Design review of the part built by this model. Coordinates are the model's own, in mm. A direction names the side the tool comes from. Give positions to 0.01 mm unless a question says otherwise; leave off trailing zeros. Loops run counter-clockwise (first coordinate to the right, second up) from the corner with the lowest first, then second, coordinate; pieces in that order, holes last. Notation, with made-up numbers: (36, 67.5) - (91, 67.5) arc R37 cw to (91, 103.5) - close; hole circle Ø11 at (-19.5, -35). An arc over 180 degrees is marked (long way). Write each question's results on one line, items separated by ' | '.
```python
from build123d import *

# Parameters (mm, degrees)
F1_DEPTH = 165.1
F3_D     = 25.4
F3_DEPTH = 25.4
F3_TIP   = 7.6309298617


with BuildPart() as f1:
    # F0 (on Right) → F1 (new body)
    with BuildSketch(Plane.YZ):
        Polygon((0, 31.75), (0, 0), (19.05, 0), (19.05, 12.7), (19.05, 31.75), align=None)
        Polygon((19.05, 31.75), (19.05, 12.7), (69.85, 12.7), (69.85, 31.75), (69.85, 44.45), (19.05, 44.45), align=None)
        Polygon((69.85, 12.7), (69.85, 0), (88.9, 0), (88.9, 31.75), (69.85, 31.75), align=None)
    extrude(amount=F1_DEPTH)

    # F3
    with Locations(Plane.XY.offset(44.45)):
        with Locations((130.302, 44.45), (35.052, 44.45)):
            Hole(F3_D / 2, depth=F3_DEPTH)
            with Locations((0, 0, -(F3_DEPTH + F3_TIP / 2))):  # 118° drill point
                Cone(0, F3_D / 2, F3_TIP, mode=Mode.SUBTRACT)


solid = f1.part
```
Item 1: Tool access review of faces 5 (the face through (81, 80, 31.75)), 6 (the face through (29.192, 33.183, 31.572)), 7 (the face through (81, 88.9, 16)), 8 (the face through (81, 10, 31.75)), 9 (the face through (81, 69.85, 6)): name each direction out of +Z, -Z, +X, -X, +Y, -Y from which nothing blocks a thin tool from reaching the whole face with its end or side.
Output values:
face 5: +Z, +X, -X, +Y | face 6: +Z | face 7: +Z, -Z, +X, -X, +Y | face 8: +Z, +X, -X, -Y | face 9: -Z, +X, -X
Item 2: Wall thickness on probe 1 along X at (y, z) = (44.45, 30.75); probe 2 along X at (y, z) = (44, 25); probe 3 along Y at (x, z) = (13, 5.5): over which ranges is each line inside the solid? List them lowest first.
Output values:
probe 1: x = 0 to 22.35, 47.75 to 117.6, 143 to 165.1 | probe 2: x = 0 to 22.36, 47.74 to 117.61, 142.99 to 165.1 | probe 3: y = 0 to 19.05, 69.85 to 88.9
Item 3: We need section D-D on x = 102.5. Give the boundary of the cut face in (y, z).
Output values:
outline: (0, 0) - (19.05, 0) - (19.05, 12.7) - (69.85, 12.7) - (69.85, 0) - (88.9, 0) - (88.9, 31.75) - (69.85, 31.75) - (69.85, 44.45) - (19.05, 44.45) - (19.05, 31.75) - (0, 31.75) - close
Item 4: We need section B-B on y = 44.45. Give the boundary of the cut face in (x, z).
Output values:
outline: (0, 12.7) - (32.92, 12.7) - (22.35, 19.05) - (22.35, 44.45) - (0, 44.45) - close; (37.18, 12.7) - (128.17, 12.7) - (117.6, 19.05) - (117.6, 44.45) - (47.75, 44.45) - (47.75, 19.05) - close; (132.43, 12.7) - (165.1, 12.7) - (165.1, 44.45) - (143, 44.45) - (143, 19.05) - close
Item 5: Draft analysis for pull direction X (two halves, no side actions). For faces 1 (the face through (34.688, 47.219, 13.097)), 2 (the face through (118.57, 39.59, 31.57)), 3 (the face through (81, 79, 0)), 4 (the face through (0, 44, 23)), state which applies: +X half, -X half, draft (parallel to the pull), parting line (faces both ways), or undercut.
Output values:
face 1: undercut | face 2: undercut | face 3: draft | face 4: -X half
Item 6: We need section C-C on z = 26.5. Give the boundary of the cut face in (x, y).
Output values:
outline: (0, 0) - (165.1, 0) - (165.1, 88.9) - (0, 88.9) - close; hole circle Ø25.4 at (35.05, 44.45); hole circle Ø25.4 at (130.3, 44.45)
Item 7: We need section A-A on z = 7. Give the boundary of the cut face in (x, y).
Output values:
outline: (0, 0) - (165.1, 0) - (165.1, 19.05) - (0, 19.05) - close; (0, 69.85) - (165.1, 69.85) - (165.1, 88.9) - (0, 88.9) - close
Item 8: Clearance check with flat-ended pins moving along their axes: P1, Ø15, axis at x = 119, y = 77.5, coming from the +Z side; P2, Ø3, axis at y = 66, z = 18, coming from the -X side; P3, Ø3, axis at y = 72, z = 36, coming from the -X side; P4, Ø10, axis at x = 72.5, z = 37, coming from the -Y side. State where each tip first meets the part, or that it passes through.
Output values:
P1: stops at z = 31.75 | P2: stops at x = 0 | P3: passes through | P4: stops at y = 19.05
